The listing builds one solid part. Answer for the finished solid, in the listing's coordinates (mm). A direction names the side the tool comes from. Coordinates: 2 decimals unless noted, no trailing zeros. Loops run counter-clockwise (first coordinate to the right, second up) from the corner with the lowest first, then second, coordinate; pieces in that order, holes last. Notation, with made-up numbers: (27, 51.5) - (33, 51.5) arc R24 ccw to (33, 67.5) - close; hole circle Ø1 at (68, 60.25). An arc over 180 degrees is marked (long way). Use one line per item in the form item = value. Start each with the question number.
```python
from build123d import *

# Parameters (mm, degrees)
F0_W     = 38.1
F0_H     = 25.4
F1_DEPTH = 2
F2_W     = 2
F2_H     = 25.4
F3_DEPTH = 2
F4_W     = 1
F4_H     = 25.4
F5_DEPTH = 1


with BuildPart() as f1:
    # F0 (on Top) → F1 (new body)
    with BuildSketch(Plane.XY):
        with Locations((1.353553, -0.729692)):
            Rectangle(F0_W, F0_H)
    extrude(amount=F1_DEPTH)

    # F2 (on face) → F3 (join)
    with BuildSketch(Plane.XY.offset(2)):
        with Locations((19.403553, -0.729692)):
            Rectangle(F2_W, F2_H)
    extrude(amount=F3_DEPTH)

    # F4 (on face) → F5 (cut)
    with BuildSketch(Plane(origin=(0, 0, 0), x_dir=(1, 0, 0), z_dir=(0, 0, -1))):
        with Locations((-16.196447, 0.729692)):
            Rectangle(F4_W, F4_H)
    extrude(amount=-F5_DEPTH, mode=Mode.SUBTRACT)


solid = f1.part
```
(1) Each of these flat-tipped pins is pushed along its axis until it touches: pin 1 Ø1.6 at (y, z) = (0, 3) entering from -X; pin 2 Ø5 at (x, y) = (2.5, 2) entering from +Z. Where does it stop, or does it pass through?
(2) For faces 1 (the face through (19, -1, 4)), 2 (the face through (18.404, -1, 3)), 3 (the face through (-16.696, -0.6, 0.5)), determine the directions among +Z, -Z, +X, -X, +Y, -Y from which every point of the face is accessible in a straight line to the end or side of a thin tool.
(3) A cutting plane is placed at C-C (x = 15). Determine the outline of the cut face in (y, z), then the cut area to 3 significant figures.
(4) A cutting plane is placed at B-B (y = -6). Determine the outline of the cut face in (x, z), then the cut area to 3 significant figures.
(5) Find the intervals of material crossed by probe 1 along X at (y, z) = (-9, 0.55); probe 2 along X at (y, z) = (3.75, 3.15); probe 3 along Z at (x, y) = (-11, 4), in increasing order. Write a range as from..to.
(6) A cutting plane is placed at D-D (z = 3.6). Determine the outline of the cut face in (x, y), then the cut area to 3 significant figures.
(7) A cutting plane is placed at A-A (z = 0.5). Determine the outline of the cut face in (x, y), then the cut area to 3 significant figures.
Evaluation:
q1.pin_1 = 18.4
q1.pin_2 = 2
q2.face_1 = +Z, +X, -X, +Y, -Y
q2.face_2 = +Z, -X, +Y, -Y
q2.face_3 = -Z, +Y, -Y
q3.outline = (-13.43, 0) - (11.97, 0) - (11.97, 2) - (-13.43, 2) - close
q3.area = 50.8 mm^2
q4.outline = (-17.7, 0) - (-16.7, 0) - (-16.7, 1) - (-15.7, 1) - (-15.7, 0) - (20.4, 0) - (20.4, 4) - (18.4, 4) - (18.4, 2) - (-17.7, 2) - close
q4.area = 79.2 mm^2
q5.probe_1 = -17.7..-16.7, -15.7..20.4
q5.probe_2 = 18.4..20.4
q5.probe_3 = 0..2
q6.outline = (18.4, -13.43) - (20.4, -13.43) - (20.4, 11.97) - (18.4, 11.97) - close
q6.area = 50.8 mm^2
q7.outline = (-17.7, -13.43) - (-16.7, -13.43) - (-16.7, 11.97) - (-17.7, 11.97) - close; (-15.7, -13.43) - (20.4, -13.43) - (20.4, 11.97) - (-15.7, 11.97) - close
q7.area = 942 mm^2
